Verification items for the finished model (mm, model axes). Face numbers are marked on the shaded views. A direction names the side the tool comes from. Coordinates: 2 decimals unless noted, no trailing zeros. Order: outer loops, then holes, each group sorted by start corner. A loop starts at its lowest first (then second) coordinate and runs counter-clockwise, first axis right, second up. Notation, with made-up numbers: M 84.25,47.5 L 101.25,47.5 A27 cw 101.25,68.5 Z; hole C 51,79.25 d5. An arc over 180 degrees is marked long. Answer as a JSON object with one key per item and string values. Group by question number.
(1) Cross-section at D-D (y = -14.75). Enter the section's corners in (x, z), plus the area to 3 significant figures.
(2) Cross-section at C-C (x = -1). Enter the section's corners in (y, z), plus the area to 3 significant figures.
(3) Gauge pin test, flat ends, axial feed: pin 1 Ø3 at (x, z) = (1, 19.5) entering from +Y; pin 2 Ø4 at (x, y) = (1, -2) entering from +Z; pin 3 Ø11.5 at (x, y) = (9.5, -8.5) entering from -Z. Record the tip position at first contact, or that the pin passes through.
(4) Cross-section at A-A (y = -1). Enter the section's corners in (x, z), plus the area to 3 significant figures.
(5) Cross-section at B-B (z = 28). Enter the section's corners in (x, y), plus the area to 3 significant figures.
(6) Access from +Z, -Z, +X, -X, +Y, -Y to the whole of each face (thin tool, end or side, straight path). Record for the marked faces 1, 2, 3 and 4.
(7) Material ranges on line 1 (Z direction, x = 1.5, y = -0.5); line 2 (Z direction, x = 4.5, y = -17); line 3 (X direction, y = -14, z = 5.5), recorded low to high.
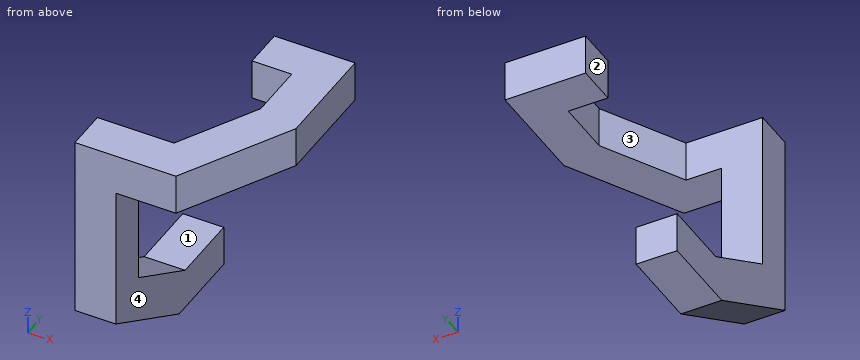
from build123d import *

# Parameters (mm, degrees)
BOSS_EXTRUDE1_DEPTH      = 2.5
BOSS_EXTRUDE1_DEPTH_BACK = 2.5
BOSS_EXTRUDE2_DEPTH      = 5


with BuildPart() as part:
    # Sketch1 → Boss-Extrude1 (new, two sides: drawn at the far end of the back side and taken through both)
    with BuildSketch(Plane(origin=(0, 0, 0), x_dir=(0, 0, -1), z_dir=(1, 0, 0)).offset(-BOSS_EXTRUDE1_DEPTH_BACK)):
        Polygon((-5, 2.397355183), (0, 2.397355183), (0, -7.568357101), (-8.160177325, -21.702198826), (-25.849658622, -21.702198826), (-25.849658622, -16.702198826), (-11.046928671, -16.702198826), (-5, -6.228611139), align=None)
    extrude(amount=BOSS_EXTRUDE1_DEPTH + BOSS_EXTRUDE1_DEPTH_BACK)

    # Sketch2 → Boss-Extrude2 (add)
    with BuildSketch(Plane.XY.offset(25.849658622)):
        Polygon((5, -16.702198826), (6.860371394, -16.702198826), (12.116424273, -6.911667965), (12.116424273, 0.006104054), (7.259579322, 0.006104054), (7.259579322, 5.006104054), (17.116424273, 5.006104054), (17.116424273, -8.168933695), (9.851082059, -21.702198826), (5, -21.702198826), (-2.5, -21.702198826), (-2.5, -16.702198826), align=None)
    extrude(amount=BOSS_EXTRUDE2_DEPTH)


solid = part.part
Taken from the geometry:
{
 "1": {"outline": "M -2.5,4.15 L 2.5,4.15 L 2.5,9.92 L -2.5,9.92 Z; M 7.91,25.85 L 13.58,25.85 L 13.58,30.85 L 7.91,30.85 Z", "area": "57.2 mm²"},
 "2": {"outline": "M -21.7,8.16 L -7.57,0 L 2.4,0 L 2.4,5 L -6.23,5 L -16.7,11.05 L -16.7,30.85 L -21.7,30.85 Z", "area": "224 mm²"},
 "3": {"pin 1": "stops at y = -16.7", "pin 2": "stops at z = 5", "pin 3": "stops at z = 25.85"},
 "4": {"outline": "M -2.5,0 L 2.5,0 L 2.5,5 L -2.5,5 Z; M 12.12,25.85 L 17.12,25.85 L 17.12,30.85 L 12.12,30.85 Z", "area": "50.0 mm²"},
 "5": {"outline": "M -2.5,-21.7 L 9.85,-21.7 L 17.12,-8.17 L 17.12,5.01 L 7.26,5.01 L 7.26,0.01 L 12.12,0.01 L 12.12,-6.91 L 6.86,-16.7 L -2.5,-16.7 Z", "area": "207 mm²"},
 "6": {"face 1": "+Z, +X, -X, +Y", "face 2": "+Z, -Z, -X, +Y", "face 3": "+Z, -Z, -X", "face 4": "-Z, +X, +Y, -Y"},
 "7": {"line 1": "z = 0 to 5", "line 2": "z = 25.85 to 30.85", "line 3": "x = -2.5 to 2.5"}
}
